Work out the finished part from the listing and answer in its coordinate system (mm). Face numbers are marked on the shaded views. A direction names the side the tool comes from. Coordinates: 2 decimals unless noted, no trailing zeros. Write each loop counter-clockwise with the first axis right and the second up, starting at its lowest first coordinate (ties: lowest second). Pieces come first, ordered by that corner, then holes. Notation, with made-up numbers: (42, 39) - (90, 39) arc R17 ccw to (90, 68) - close; hole circle Ø6 at (13, 74). An arc over 180 degrees is marked (long way). One line per item, written item: value.
Autodesk Inventor part; units mm, degrees
ref_plane "bolt_to_nut_XY" through (4.3, 0, 0) normal (1, 0, 0) x (0, 0, -1)
ref_plane "bolt_to_nut_YZ" through (4.3, 0, 0) normal (0, 0, -1) x (0, 1, 0)
ref_plane "bolt_to_nut_ZX" through (4.3, 0, 0) normal (0, 1, 0) x (1, 0, 0)
sketch "Sketch_1" plane through (0, 0, 0) normal (0, 0, 1) x (1, 0, 0)
  line L0 (4.3, 0) -> (0, 0)
  line L1 (-1.7, 0) -> (-1.7, 3)
  line L2 (-1.7, 3) -> (-1.5, 3)
  line L3 (-1.5, 3) -> (0, 1.5)
  line L4 (0, 1.5) -> (3.9935, 1.5)
  line L5 (3.9935, 1.5) -> (4.3, 1.1935)
  line L6 (4.3, 1.1935) -> (4.3, 0)
  line L7 (4.3, 0) -> (-1.7, 0)
revolve "Revolution1" add sketch "Sketch_1" angle 360 about axis through (4.3, 0, 0) along (1, 0, 0)
thread "Thread1"
sketch "Sketch2" plane through (-1.7, 0, 0) normal (-1, 0, 0) x (0, 0, 1)
  point P0 (0, 0)
hole "Hole1" at (-1.7, 0, 0) direction (1, 0, 0) diameter 2 depth 0.85 tip angle 150
sketch "Sketch_3" plane through (-1.7, 0, 0) normal (1, 0, 0) x (0, 0, -1)
  line L0 (-1, -0.5774) -> (0, -1.1547)
  line L1 (0, -1.1547) -> (1, -0.5774)
  line L2 (1, -0.5774) -> (1, 0.5774)
  line L3 (1, 0.5774) -> (0, 1.1547)
  line L4 (0, 1.1547) -> (-1, 0.5774)
  line L5 (-1, 0.5774) -> (-1, -0.5774)
extrude "Extrusion1" cut sketch "Sketch_3" along normal blind 0.85
ref_plane "bolt_to_nut_XY" through (4.3, 0, 0) normal (1, 0, 0) x (0, 0, -1)
ref_plane "bolt_to_nut_YZ" through (4.3, 0, 0) normal (0, 0, -1) x (0, 1, 0)
ref_plane "bolt_to_nut_ZX" through (4.3, 0, 0) normal (0, 1, 0) x (1, 0, 0)
ref_plane "dummy_to_bolt_XY" through (0, 0, 0) normal (1, 0, 0) x (0, 0, -1)
ref_plane "dummy_to_bolt_YZ" through (0, 0, 0) normal (0, 0, -1) x (0, 1, 0)
ref_plane "dummy_to_bolt_ZX" through (0, 0, 0) normal (0, 1, 0) x (1, 0, 0)
properties part number "HFBCM3-6"
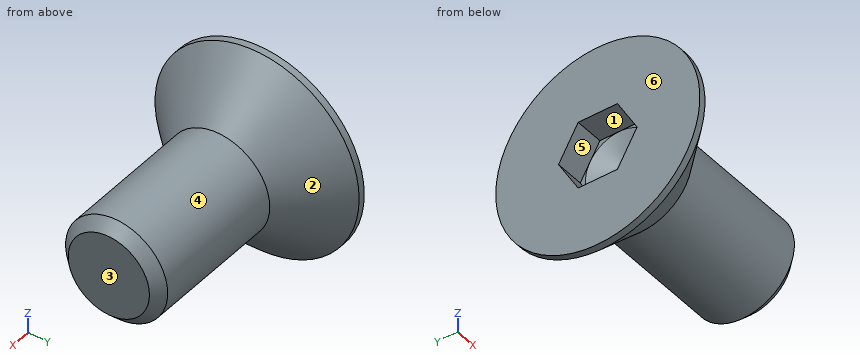
Item 1: Section A-A, the plane x = 2.95 is taken. Determine the outline of the cut face in (y, z).
Evaluation:
outline: circle Ø3 at (0, 0)
Item 2: Given pin 1 (3 mm diameter, centred on x = 2.5, z = 0.5, fed in from +Y); pin 2 (1 mm diameter, centred on x = 1.5, y = -1, fed in from -Z), each flat-ended and moving along its own axis, determine where each tip first touches the part or whether it passes through.
Evaluation:
pin 1: stops at y = 1.5
pin 2: stops at z = -1.41
Item 3: Consider probe 1 along X at (y, z) = (-2.5, 1); probe 2 along Z at (x, y) = (0.85, 0.05); probe 3 along X at (y, z) = (1.4, -1.4). Determine where each line is inside the solid, lowest interval first.
Evaluation:
probe 1: x = -1.7 to -1.19
probe 2: z = -1.5 to 1.5
probe 3: x = -1.7 to -0.48
Item 4: Which of the six approach directions +Z, -Z, +X, -X, +Y, -Y give full straight-line access (tool end or side, diameter ignored) to the marked faces 4, 5 and 6?
Evaluation:
face 4: +X
face 5: -X
face 6: +Z, -Z, -X, +Y, -Y
Item 5: Determine the mould class of the marked faces 1, 2 and 3 for opening direction Z: +Z half, -Z half, draft (parallel to the pull), parting line (faces both ways), or undercut.
Evaluation:
face 1: undercut
face 2: parting line
face 3: draft
